Work out the finished part from the listing and answer in its coordinate system (mm). A direction names the side the tool comes from. Coordinates: 2 decimals unless noted, no trailing zeros. Loops run counter-clockwise (first coordinate to the right, second up) from the corner with the lowest first, then second, coordinate; pieces in that order, holes last. Notation, with made-up numbers: (72, 77) -> (89, 77) arc R14 ccw to (89, 94) -> close; hole circle Ø4 at (47.25, 41.5). An arc over 180 degrees is marked (long way). Use a Markdown table: item, result.
from build123d import *

# Parameters (mm, degrees)
SKETCH1_R           = 1.45
SKETCH1_R_2         = 1.95
BOSS_EXTRUDE1_DEPTH = 5


with BuildPart() as part:
    # Sketch1 → Boss-Extrude1 (new body)
    with BuildSketch(Plane.XY):
        with BuildLine():
            Line((60, 30.470821026), (68.531226941, 30.470821026))
            ThreePointArc((68.531226941, 30.470821026), (74.141161233, -11.317606244), (56.31927228, -49.529178974))
            Line((56.31927228, -49.529178974), (56.31927228, -57.529178974))
            Line((56.31927228, -57.529178974), (33.865327846, -57.529178974))
            Line((33.865327846, -57.529178974), (33.865327846, -49.529178974))
            ThreePointArc((33.865327846, -49.529178974), (53.065618204, -28.000717216), (60, 0))
            Line((60, 0), (60, 30.470821026))
        make_face()
        with Locations((38.092300063, -53.529178974)):
            Circle(SKETCH1_R, mode=Mode.SUBTRACT)
        with Locations((52.092300063, -51.529178974)):
            Circle(SKETCH1_R_2, mode=Mode.SUBTRACT)
    extrude(amount=BOSS_EXTRUDE1_DEPTH)


solid = part.part
Q1. Given pin 1 Ø2.5 at (y, z) = (19.5, 3) entering from -X; pin 2 Ø2.5 at (y, z) = (-53.5, 2) entering from +X; pin 3 Ø1 at (x, z) = (38.5, 0.5) entering from +Y, each flat-ended and moving along its own axis, determine where each tip first touches the part or whether it passes through.
Solved:
| item | result |
|---|---|
| pin 1 | x = 60 |
| pin 2 | x = 56.32 |
| pin 3 | y = -45.6 |
Q2. Section C-C on x = 43.5 is taken. Determine the outline of the cut face in (y, z).
Solved:
| item | result |
|---|---|
| outline | (-57.53, 0) -> (-41.32, 0) -> (-41.32, 5) -> (-57.53, 5) -> close |
Q3. Determine the mould class of faces 4 (the cylindrical face through (37.9, -52.09, 2.46)), 5 (the flat face through (45, -57.529, 2)), 6 (the cylindrical face through (52.874, -28.361, 2.465)) for opening direction X: pulls with the +X half, pulls with the -X half, needs draft (parallel to the pull), parting line crosses it, or undercut.
Solved:
| item | result |
|---|---|
| face 4 | undercut |
| face 5 | needs draft |
| face 6 | pulls with the -X half |
Q4. Section A-A on z = 3.7 is taken. Determine the outline of the cut face in (x, y), and give its area (3 significant figures).
Solved:
| item | result |
|---|---|
| outline | (33.87, -57.53) -> (56.32, -57.53) -> (56.32, -49.53) arc R75 ccw to (68.53, 30.47) -> (60, 30.47) -> (60, 0) arc R60 cw to (33.87, -49.53) -> close; hole circle Ø2.9 at (38.09, -53.53); hole circle Ø3.9 at (52.09, -51.53) |
| area | 1,390 mm² |
Q5. Section B-B on y = -25.5 is taken. Determine the outline of the cut face in (x, z), and give its area (3 significant figures).
Solved:
| item | result |
|---|---|
| outline | (54.31, 0) -> (70.53, 0) -> (70.53, 5) -> (54.31, 5) -> close |
| area | 81.1 mm² |
Q6. For faces 1 (the flat face through (59, -13, 5)), 2 (the flat face through (60, 15, 2)), 3 (the flat face through (56.319, -53, 2)), determine the directions among +Z, -Z, +X, -X, +Y, -Y from which every point of the face is accessible in a straight line to the end or side of a thin tool.
Solved:
| item | result |
|---|---|
| face 1 | +Z, +X, -X, +Y, -Y |
| face 2 | +Z, -Z, -X, +Y |
| face 3 | +Z, -Z, +X, -Y |
Q7. Consider line 1 (Y direction, x = 39, z = 4.3); line 2 (X direction, y = -15, z = 1.05); line 3 (X direction, y = -13, z = 2.35). Determine where each line is inside the solid, lowest interval first. Write a range as [from, to].
Solved:
| item | result |
|---|---|
| line 1 | [-57.53, -54.66], [-52.4, -45.6] |
| line 2 | [58.09, 73.48] |
| line 3 | [58.57, 73.86] |
